Print and shaded views of the part. All mm, measured from the part's lowest x, y and z. A direction names the side the tool comes from. Round coordinates to 2 decimals unless told otherwise and drop trailing zeros. Write each loop counter-clockwise with the first axis right and the second up, starting at its lowest first coordinate (ties: lowest second). Pieces come first, ordered by that corner, then holes. Notation, with made-up numbers: (29, 0.5) -> (78, 0.5) arc R10 ccw to (78, 17.5) -> close; hole circle Ø3 at (42, 81). An arc over 180 degrees is marked (long way). Return JSON: item names as keys, results as strings. Group by question number.
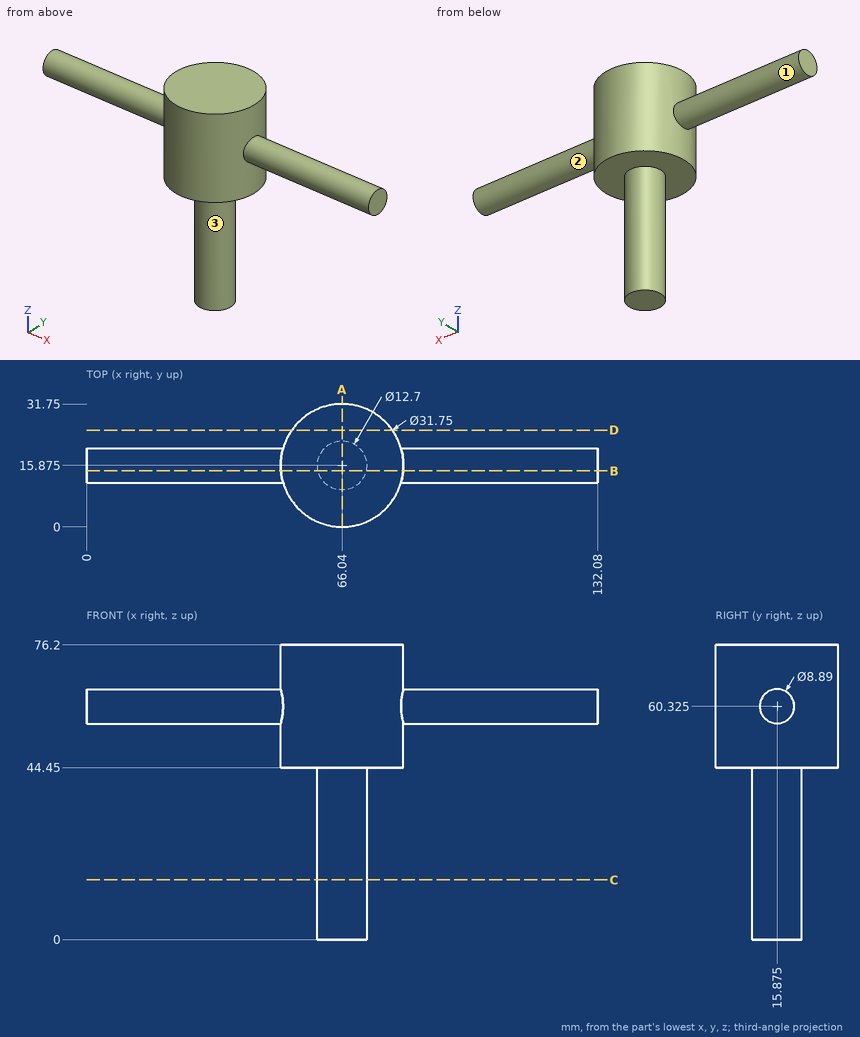
Item 1: Which spindle directions (+Z, -Z, +X, -X, +Y, -Y) get a long thin tool onto all of the face, cutting with end or side? Do the marked faces 1, 2 and 3. Say none if no direction does.
Item 2: Cut at D-D (y = 25). Write the cut outline in (x, z), then the cut area to 3 significant figures.
Item 3: Flat gauge pins, fed straight in: P1, Ø5, axis at y = 9, z = 50, coming from the +X side; P2, Ø1.5, axis at y = 25.5, z = 57.5, coming from the -X side; P3, Ø12, axis at x = 112.5, y = 9.5, coming from the +Z side. Where does each tip first touch, or does it go through?
Item 4: Cut at A-A (x = 66.04). Write the cut outline in (y, z) (3 decimals), then the cut area to 3 significant figures.
Item 5: Wall check: L1, parallel to Z at x = 73, y = 26; L2, parallel to Y at x = 16, z = 60; L3, parallel to X at y = 9.5, z = 56.5. Give the ranges that are in metal, low to high.
Item 6: Cut at C-C (z = 15.5). Write the cut outline in (x, y) (3 decimals), then the cut area to 3 significant figures.
Item 7: Cut at B-B (y = 14.5). Write the cut outline in (x, z).
Checks:
{
 "1": {"face 1": "-X", "face 2": "+X", "face 3": "-Z"},
 "2": {"outline": "(53.05, 44.45) -> (79.03, 44.45) -> (79.03, 76.2) -> (53.05, 76.2) -> close", "area": "825 mm2"},
 "3": {"P1": "stops at x = 81.3", "P2": "stops at x = 52.88", "P3": "stops at z = 64.75"},
 "4": {"outline": "(0, 44.45) -> (9.525, 44.45) -> (9.525, 0) -> (22.225, 0) -> (22.225, 44.45) -> (31.75, 44.45) -> (31.75, 76.2) -> (0, 76.2) -> close", "area": "1,570 mm2"},
 "5": {"L1": "z = 44.45 to 76.2", "L2": "y = 11.44 to 20.31", "L3": "x = 51.5 to 80.58"},
 "6": {"outline": "circle Ø12.7 at (66.04, 15.875)", "area": "127 mm2"},
 "7": {"outline": "(0, 56.1) -> (50.22, 56.1) -> (50.22, 44.45) -> (59.84, 44.45) -> (59.84, 0) -> (72.24, 0) -> (72.24, 44.45) -> (81.86, 44.45) -> (81.86, 56.1) -> (132.08, 56.1) -> (132.08, 64.55) -> (81.86, 64.55) -> (81.86, 76.2) -> (50.22, 76.2) -> (50.22, 64.55) -> (0, 64.55) -> close"}
}
